from build123d import *

# Parameters (mm, degrees)
BOX001_W          = 30
BOX001_H          = 70
BOX001_DEPTH      = 10
CYLINDER003_R     = 5
CYLINDER003_DEPTH = 40
CYLINDER002_R     = 18.5
CYLINDER002_DEPTH = 25


with BuildPart() as cube001:
    # Box001 → Box001 (new body)
    with BuildSketch(Plane(origin=(7.5, -20, 9), x_dir=(1, 0, 0), z_dir=(0, 0, 1))):
        with Locations((15, 35)):
            Rectangle(BOX001_W, BOX001_H)
    extrude(amount=BOX001_DEPTH)


with BuildPart() as cylinder003:
    # Cylinder003 → Cylinder003 (new body)
    with BuildSketch(Plane.XY.offset(-10)):
        Circle(CYLINDER003_R)
    extrude(amount=CYLINDER003_DEPTH)


with BuildPart() as mount:
    # Cylinder002 → Cylinder002 (new body)
    with BuildSketch(Plane.XY):
        Circle(CYLINDER002_R)
    extrude(amount=CYLINDER002_DEPTH)

    # Cut002: cut Cylinder003
    add(cylinder003.part, mode=Mode.SUBTRACT)

    # Cut003: cut Cube001
    add(cube001.part, mode=Mode.SUBTRACT)


solid = mount.part
Model file for the job. Use its own axes, mm. A direction names the side the tool comes from. Give positions to 0.01 mm unless a question says otherwise; leave off trailing zeros. Write each loop counter-clockwise with the first axis right and the second up, starting at its lowest first coordinate (ties: lowest second). Pieces come first, ordered by that corner, then holes. Notation, with made-up numbers: (60, -0.5) - (94, -0.5) arc R25 cw to (94, 17.5) - close; hole circle Ø6 at (74.25, -22). An arc over 180 degrees is marked (long way). Answer as CSV lines item,"result".
1. Band-saw the part on B-B (x = 0). Write the cut outline in (y, z), and give its area (3 significant figures).
Responses:
outline,"(-18.5, 0) - (-5, 0) - (-5, 25) - (-18.5, 25) - close; (5, 0) - (18.5, 0) - (18.5, 25) - (5, 25) - close"
area,"675 mm2"
2. Two-plate mould, pull along Z, no slides. Class faces 3 (the face through (7.5, 0, 14)), 4 (the face through (-1.08, -4.88, 12.32)), 5 (the face through (12, 0, 9)), 6 (the face through (4, -4, 0)): +Z half, -Z half, draft (parallel to the pull), parting line (faces both ways), or undercut.
Responses:
face 3,"undercut"
face 4,"draft"
face 5,"undercut"
face 6,"-Z half"
3. Drill centre lines: L1, parallel to Y at x = 0, z = 5; L2, parallel to X at y = -7.5, z = 11.5; L3, parallel to X at y = 1, z = 7.5. Where is each one in solid material? Low to high. Write a range as [from, to].
Responses:
L1,"y = [-18.5, -5], [5, 18.5]"
L2,"x = [-16.91, 7.5]"
L3,"x = [-18.47, -4.9], [4.9, 18.47]"
4. 3-axis set-ups, long thin cutter, end or side, ignore diameter. For faces 1 (the face through (-18.482, 0.813, 12.325)), 2 (the face through (12, 0, 19)): which of +Z, -Z, +X, -X, +Y, -Y reach the whole face in a straight line?
Responses:
face 1,"+Z, -Z"
face 2,"+X, +Y, -Y"
5. Band-saw the part on D-D (y = -11.5). Write the cut outline in (x, z).
Responses:
outline,"(-14.49, 0) - (14.49, 0) - (14.49, 9) - (7.5, 9) - (7.5, 19) - (14.49, 19) - (14.49, 25) - (-14.49, 25) - close"
6. Band-saw the part on A-A (y = 0). Write the cut outline in (x, z).
Responses:
outline,"(-18.5, 0) - (-5, 0) - (-5, 25) - (-18.5, 25) - close; (5, 0) - (18.5, 0) - (18.5, 9) - (7.5, 9) - (7.5, 19) - (18.5, 19) - (18.5, 25) - (5, 25) - close"
7. Band-saw the part on C-C (z = 16.25). Write the cut outline in (x, y), and give its area (3 significant figures).
Responses:
outline,"(7.5, -16.91) - (7.5, 16.91) arc R18.5 ccw (long way) to start; hole circle Ø10 at (0, 0)"
area,"729 mm2"
8. Pin check, flat tips, straight feed: pin 1 (3 mm diameter, centred on y = -4, z = 12.5, fed in from +X); pin 2 (2 mm diameter, centred on y = -1.5, z = 20.5, fed in from +X); pin 3 (5 mm diameter, centred on y = -7, z = 8.5, fed in from -X). Stop position of each tip, or through.
Responses:
pin 1,"stops at x = 7.5"
pin 2,"stops at x = 18.49"
pin 3,"stops at x = -17.94"
